from build123d import *

# Parameters (mm, degrees)
F0_R     = 4.7625
F1_DEPTH = 19.05


# Not quite as in the source:
# - ends of sketch curves that miss each other by under 0.0002 mm in the source are joined


with BuildPart() as f1:
    # F0 (on Top) → F1 (new body)
    with BuildSketch(Plane.XY):
        with BuildLine():
            Line((-221.8857894, -106.4373771847), (-221.8857894, -88.1065191612))
            Line((-221.8857894, -88.1065191612), (-231.0306276, -82.826733))
            ThreePointArc((-231.0306276, -82.826733), (-238.3890078323, -75.1524401819), (-240.4883816501, -64.7297166236))
            ThreePointArc((-240.4883816501, -64.7297166236), (-248.2560543221, -26.1655958132), (-275.4820809487, 2.2293229893))
            ThreePointArc((-275.4820809487, 2.2293229893), (-297.7142880041, 10.461378966), (-321.4183295937, 10.8565858382))
            ThreePointArc((-321.4183295937, 10.8565858382), (-327.8248357317, 10.9634065797), (-333.8335467811, 13.1882885934))
            Line((-333.8335467811, 13.1882885934), (-362.314236, 29.6316146))
            Line((-362.314236, 29.6316146), (-413.114236, -58.3565508))
            Line((-413.114236, -58.3565508), (-384.6335462, -74.7999012))
            ThreePointArc((-384.6335462, -74.7999012), (-379.7023894379, -78.8911519852), (-376.4066376642, -84.3859370356))
            ThreePointArc((-376.4066376642, -84.3859370356), (-364.2123588019, -104.7166445735), (-345.9670808498, -119.8542782393))
            ThreePointArc((-345.9670808498, -119.8542782393), (-307.7633473097, -129.2352495129), (-270.4820087562, -116.6801838382))
            ThreePointArc((-270.4820087562, -116.6801838382), (-260.4059713642, -113.286900565), (-250.0806270189, -115.8222971934))
            Line((-250.0806270189, -115.8222971934), (-237.760637, -122.9352634))
            ThreePointArc((-237.760637, -122.9352634), (-232.9421342351, -123.569614107), (-229.0863779145, -120.6109894599))
            Line((-229.0863779145, -120.6109894599), (-224.3238846, -112.362107))
            Line((-224.3238846, -112.362107), (-273.3642488, -84.0486254))
            ThreePointArc((-273.3642488, -84.0486254), (-281.1433177605, -92.8360964437), (-290.9268252362, -99.3181139076))
            ThreePointArc((-290.9268252362, -99.3181139076), (-292.2425670349, -100.5162816603), (-292.7069827203, -102.2341617784))
            ThreePointArc((-292.7069827203, -102.2341617784), (-297.4122125633, -108.4948669165), (-304.6174116153, -105.4255515302))
            ThreePointArc((-304.6174116153, -105.4255515302), (-305.8785439427, -104.1700351993), (-307.6170882048, -103.7902477201))
            ThreePointArc((-307.6170882048, -103.7902477201), (-333.2670739258, -97.8572369807), (-351.2302185284, -78.6102104616))
            ThreePointArc((-351.2302185284, -78.6102104616), (-352.4283762603, -77.2944637651), (-354.1462563784, -76.8300480797))
            ThreePointArc((-354.1462563784, -76.8300480797), (-360.4069615165, -72.1248182367), (-357.3376461302, -64.9196191847))
            ThreePointArc((-357.3376461302, -64.9196191847), (-356.0821208015, -63.6584957522), (-355.7023440666, -61.9199427159))
            ThreePointArc((-355.7023440666, -61.9199427159), (-349.7693252458, -36.2699713018), (-330.5223050616, -18.3068376716))
            ThreePointArc((-330.5223050616, -18.3068376716), (-329.2065612709, -17.1086592996), (-328.7421426797, -15.3907744216))
            ThreePointArc((-328.7421426797, -15.3907744216), (-324.0369128367, -9.1300692835), (-316.8317137847, -12.1993846698))
            ThreePointArc((-316.8317137847, -12.1993846698), (-315.5705903522, -13.4549099985), (-313.8320373159, -13.8346867334))
            ThreePointArc((-313.8320373159, -13.8346867334), (-288.1820750251, -19.7677256868), (-270.2189422924, -39.0147306362))
            ThreePointArc((-270.2189422924, -39.0147306362), (-269.0207538996, -40.3304695291), (-267.3028690216, -40.7948881203))
            ThreePointArc((-267.3028690216, -40.7948881203), (-261.0421638835, -45.5001179633), (-264.1114792698, -52.7053170153))
            ThreePointArc((-264.1114792698, -52.7053170153), (-265.3669956007, -53.9664493427), (-265.7467830799, -55.7049936048))
            ThreePointArc((-265.7467830799, -55.7049936048), (-266.4686255378, -67.4187649457), (-270.1892527015, -78.5493711003))
            Line((-270.1892527015, -78.5493711003), (-221.8857894, -106.4373771847))
        make_face()
        with Locations((-339.6170754, -108.8557386)):
            Circle(F0_R, mode=Mode.SUBTRACT)
        with Locations((-281.8320754, -8.7691976)):
            Circle(F0_R, mode=Mode.SUBTRACT)
        with BuildLine():
            Line((-218.710637, -89.9396982), (-221.8857894, -88.1065191612))
            Line((-221.8857894, -88.1065191612), (-221.8857894, -106.4373771847))
            Line((-221.8857894, -106.4373771847), (-221.1488846, -106.8628292))
            Line((-221.1488846, -106.8628292), (-216.3863846, -98.6139506))
            ThreePointArc((-216.3863846, -98.6139506), (-215.7520068495, -93.7954539688), (-218.710637, -89.9396982))
        make_face()
    extrude(amount=F1_DEPTH)


solid = f1.part
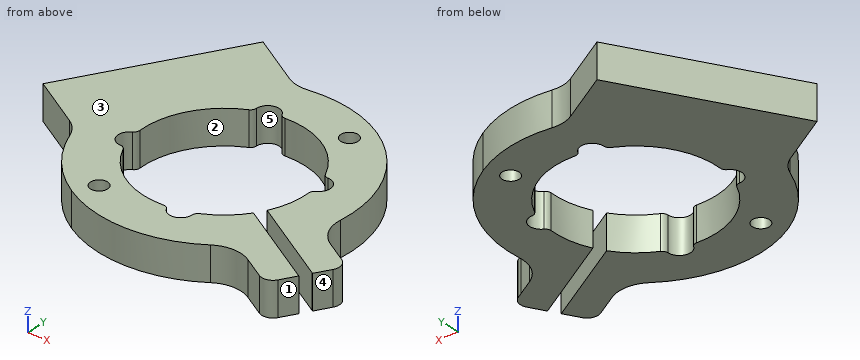
Read the model definition and answer for the solid it produces. Units are mm, in the model's axes. Face numbers are marked on the shaded views. A direction names the side the tool comes from. Round coordinates to 2 decimals unless told otherwise and drop trailing zeros. Loops run counter-clockwise (first coordinate to the right, second up) from the corner with the lowest first, then second, coordinate; pieces in that order, holes last. Notation, with made-up numbers: (-9, -34) - (18, -34) arc R25 cw to (18, -7) - close; hole circle Ø1 at (13, -34.5). An arc over 180 degrees is marked (long way). One line per question, with ' | ' between items. Start each with the question number.
Q1. Section C-C on z = 8.5 is taken. Count the separate pieces of the cut face and the enclosed holes in it, plus the area to 3 significant figures.
Q2. For the marked faces 1 and 2, determine the directions among +Z, -Z, +X, -X, +Y, -Y from which every point of the face is accessible in a straight line to the end or side of a thin tool.
Q3. Find the intervals of material crossed by L1, parallel to Y at x = -279, z = 5; L2, parallel to Y at x = -285.5, z = 1; L3, parallel to X at y = -88.5, z = 6.5, in increasing order.
Q4. For a pull along X with two mould halves and no side action, classify the marked faces 3, 4 and 5 as +X half, -X half, draft (parallel to the pull), parting line (faces both ways), or undercut.
Q5. Flat-ended cylindrical pins translate along their axes: pin 1 (6 mm diameter, centred on x = -284.5, z = 9, fed in from -Y); pin 2 (5 mm diameter, centred on y = -101, z = 8.5, fed in from -X); pin 3 (10 mm diameter, centred on y = 7.5, z = 7, fed in from -X); pin 4 (4 mm diameter, centred on x = -257, y = -45.5, fed in from -Z). Find the tip coordinate at first contact, or state that the pin passes through.
Q6. Section D-D on x = -284.5 is taken. Give the vertices of the cut face in (y, z).
Q7. Section B-B on y = -50 is taken. Give the vertices of the cut face in (x, z).
Q8. Section A-A on x = -339.5 is taken. Give the vertices of the cut face in (y, z).
Established:
1) separate pieces: 1 | enclosed holes: 2 | area: 12,300 mm²
2) face 1: +Z, -Z, +X, -Y | face 2: +Z, -Z
3) L1: -121.75 to -90.85, -26.78 to -12.6, -4.94 to 4.13 | L2: -124.63 to -96.18, -21.44 to -11.81, -5.73 to 7 | L3: -374.65 to -344.66, -276.79 to -265.65, -252.95 to -221.2
4) face 3: draft | face 4: +X half | face 5: undercut
5) pin 1: y = -125.36 | pin 2: x = -368.97 | pin 3: x = -377.98 | pin 4: z = 0
6) outline: (-124.24, 0) - (-95.49, 0) - (-95.49, 19.05) - (-124.24, 19.05) - close; (-22.14, 0) - (-12.71, 0) - (-12.71, 19.05) - (-22.14, 19.05) - close; (-4.82, 0) - (6.61, 0) - (6.61, 19.05) - (-4.82, 19.05) - close
7) outline: (-408.29, 0) - (-354.94, 0) - (-354.94, 19.05) - (-408.29, 19.05) - close; (-261.5, 0) - (-240.79, 0) - (-240.79, 19.05) - (-261.5, 19.05) - close
8) outline: (-123.16, 0) - (-113.62, 0) - (-113.62, 19.05) - (-123.16, 19.05) - close; (-104.09, 0) - (-93.52, 0) - (-93.52, 19.05) - (-104.09, 19.05) - close; (-24.1, 0) - (16.46, 0) - (16.46, 19.05) - (-24.1, 19.05) - close
